Design review of the part built by this model. Coordinates are the model's own, in mm. A direction names the side the tool comes from. Round coordinates to 2 decimals unless told otherwise and drop trailing zeros. Write each loop counter-clockwise with the first axis right and the second up, starting at its lowest first coordinate (ties: lowest second). Pieces come first, ordered by that corner, then holes. Notation, with made-up numbers: (32.5, 40.5) - (66.5, 40.5) arc R24 cw to (66.5, 78.5) - close; hole circle Ø6 at (15, 54.5). An arc over 180 degrees is marked (long way). Use one line per item in the form item = value.
```python
from build123d import *

# Parameters (mm, degrees)
F2_R     = 4.7752
F3_DEPTH = 11.43
F4_R     = 1.59258
F5_DEPTH = 19.685


with BuildPart() as f1:
    # F0 (on Front) → F1 (revolve)
    with BuildSketch(Plane.XZ):
        with BuildLine():
            Line((0, 49.53), (0, 0))
            Line((0, 0), (7.62, 4.5790501198))
            add(Edge.make_bspline(
                [(7.62, 4.5790501198), (29.7629128184, 6.2660863931), (38.3151381872, 16.6933844429), (-7.2643313704, 19.7713115256), (36.777698875, 22.9889912098), (6.7876640157, 29.4968915755), (7.4576054123, 30.2991130403), (7.62, 30.48)],
                knots=[0, 0, 0, 0, 0.264066964, 0.5177980437, 0.7376172199, 0.9619915978, 1, 1, 1, 1], degree=3))
            Line((7.62, 30.48), (7.62, 49.53))
            Line((7.62, 49.53), (0, 49.53))
        make_face()
    revolve(axis=Axis((0, 0, 24.765), (0, 0, -1)))

    # F2 (on face) → F3 (cut)
    with BuildSketch(Plane.XY.offset(49.53)):
        Circle(F2_R)
    extrude(amount=-F3_DEPTH, mode=Mode.SUBTRACT)

    # F4 (on Top) → F5 (cut)
    with BuildSketch(Plane.XY):
        Circle(F4_R)
    extrude(amount=F5_DEPTH, mode=Mode.SUBTRACT)


solid = f1.part
```
Q1. We need section A-A on z = 42. Write out the cut boundary in (x, y).
Calculated:
outline = circle Ø15.24 at (0, 0); hole circle Ø9.55 at (0, 0)
Q2. For P1, Ø10, axis at y = 15, z = 26, coming from the +X side; P2, Ø5, axis at x = -0.5, z = 16, coming from the +Y side; P3, Ø12, axis at x = 3, y = 21, coming from the +Z side, all flat-tipped, find the tip position at first contact; note any pin that passes through.
Calculated:
P1 = 20.36
P2 = 29.72
P3 = 27.56
Q3. To check wall thickness, follow line 1 along Y through (x, z) = (0, 42); line 2 along Y through (x, z) = (0, 12); line 3 along Z through (x, y) = (-3, -10). State the ranges of each line that lie inside material, in increasing order. Write a range as from..to.
Calculated:
line_1 = -7.62..-4.78, 4.78..7.62
line_2 = -30.49..-1.59, 1.59..30.49
line_3 = 4.82..18.9, 20.72..28.99
Q4. Machinability: for faces 1 (the cylindrical face through (-1.65, 7.44, 40.14)), 2 (the cylindrical face through (1.52, 0.48, 10.19)), which of the approach directions +Z, -Z, +X, -X, +Y, -Y give a long, thin tool a straight path to every point of the face, cutting with its end or side? Answer none if there is none.
Calculated:
face_1 = +Z
face_2 = -Z
Q5. Draft analysis for pull direction X (two halves, no side actions). For faces 3 (the flat face through (0, 0, 38.1)), 4 (the conical face through (1.879, -0.592, 1.184)), 5 (the flat face through (0, 5, 49.53)), 6 (the flat face through (0, 0, 19.685)), state which applies: released by +X, released by -X, zero draft, split by the parting line, or undercut.
Calculated:
face_3 = undercut
face_4 = split by the parting line
face_5 = zero draft
face_6 = undercut
